Geometry: final body of the model. Coordinates: model frame, mm. A direction names the side the tool comes from. Give positions to 0.01 mm unless a question says otherwise; leave off trailing zeros. Write each loop counter-clockwise with the first axis right and the second up, starting at its lowest first coordinate (ties: lowest second). Pieces come first, ordered by that corner, then holes.
```python
from build123d import *

# Parameters (mm, degrees)
CYLINDER027_R     = 2
CYLINDER027_DEPTH = 10
CYLINDER025_R     = 2
CYLINDER025_DEPTH = 10
CYLINDER024_R     = 2
CYLINDER024_DEPTH = 10
CYLINDER023_R     = 4
CYLINDER023_DEPTH = 60
CYLINDER028_R     = 7.5
CYLINDER028_DEPTH = 40
BOX005_W          = 25
BOX005_H          = 25
BOX005_DEPTH      = 5.2


with BuildPart() as cylinder027:
    # Cylinder027 → Cylinder027 (new body)
    with BuildSketch(Plane(origin=(21, 4, -2), x_dir=(1, 0, 0), z_dir=(0, 0, 1))):
        Circle(CYLINDER027_R)
    extrude(amount=CYLINDER027_DEPTH)


with BuildPart() as cylinder025:
    # Cylinder025 → Cylinder025 (new body)
    with BuildSketch(Plane(origin=(4, 21, -2), x_dir=(1, 0, 0), z_dir=(0, 0, 1))):
        Circle(CYLINDER025_R)
    extrude(amount=CYLINDER025_DEPTH)


with BuildPart() as cylinder024:
    # Cylinder024 → Cylinder024 (new body)
    with BuildSketch(Plane(origin=(4, 4, -2), x_dir=(1, 0, 0), z_dir=(0, 0, 1))):
        Circle(CYLINDER024_R)
    extrude(amount=CYLINDER024_DEPTH)


with BuildPart() as cylinder023:
    # Cylinder023 → Cylinder023 (new body)
    with BuildSketch(Plane(origin=(12.5, 12.5, -7), x_dir=(1, 0, 0), z_dir=(0, 0, 1))):
        Circle(CYLINDER023_R)
    extrude(amount=CYLINDER023_DEPTH)


with BuildPart() as cylinder028:
    # Cylinder028 → Cylinder028 (new body)
    with BuildSketch(Plane(origin=(12.5, 12.5, 5), x_dir=(1, 0, 0), z_dir=(0, 0, 1))):
        Circle(CYLINDER028_R)
    extrude(amount=CYLINDER028_DEPTH)


with BuildPart() as cut026:
    # Box005 → Box005 (new body)
    with BuildSketch(Plane.XY):
        with Locations((12.5, 12.5)):
            Rectangle(BOX005_W, BOX005_H)
    extrude(amount=BOX005_DEPTH)

    # Fusion006: union Cylinder028
    add(cylinder028.part)

    # Cut027: cut Cylinder023
    add(cylinder023.part, mode=Mode.SUBTRACT)

    # Cut028: cut Cylinder024
    add(cylinder024.part, mode=Mode.SUBTRACT)

    # Cut025: cut Cylinder025
    add(cylinder025.part, mode=Mode.SUBTRACT)

    # Cut026: cut Cylinder027
    add(cylinder027.part, mode=Mode.SUBTRACT)


solid = cut026.part
```
Item 1: Section D-D, the plane z = 7.5. Return the cut outline in (x, y), plus the area to 3 significant figures.
Found:
outline: circle Ø15 at (12.5, 12.5); hole circle Ø8 at (12.5, 12.5)
area: 126 mm2
Item 2: Pull-direction query (X, two-part tool) for faces 1 (the face through (11.979, 16.466, 22.185)), 2 (the face through (12, 25, 3)), 3 (the face through (0, 12, 3)); classes: +X half, -X half, draft (parallel to the pull), parting line (faces both ways), or undercut.
Found:
face 1: undercut
face 2: draft
face 3: -X half
Item 3: Section C-C, the plane y = 21. Return the cut outline in (x, z).
Found:
outline: (0, 0) - (2, 0) - (2, 5.2) - (0, 5.2) - close; (6, 0) - (25, 0) - (25, 5.2) - (6, 5.2) - close
Item 4: Line query: L1, parallel to Y at x = 4, z = 4; L2, parallel to X at y = 12.5, z = 15.5. Output: solid intervals per line, ascending.
Found:
L1: y = 0 to 2, 6 to 19, 23 to 25
L2: x = 5 to 8.5, 16.5 to 20
Item 5: Section A-A, the plane x = 12.5. Return the cut outline in (y, z), plus the area to 3 significant figures.
Found:
outline: (0, 0) - (8.5, 0) - (8.5, 45) - (5, 45) - (5, 5.2) - (0, 5.2) - close; (16.5, 0) - (25, 0) - (25, 5.2) - (20, 5.2) - (20, 45) - (16.5, 45) - close
area: 367 mm2
Item 6: Section B-B, the plane y = 4. Return the cut outline in (x, z), plus the area to 3 significant figures.
Found:
outline: (0, 0) - (2, 0) - (2, 5.2) - (0, 5.2) - close; (6, 0) - (19, 0) - (19, 5.2) - (6, 5.2) - close; (23, 0) - (25, 0) - (25, 5.2) - (23, 5.2) - close
area: 88.4 mm2
Item 7: Reachability of faces 4 (the face through (10.87, 5.18, 24.82)), 5 (the face through (19.4, 2.8, 2.6)) from +Z, -Z, +X, -X, +Y, -Y: full face, straight path, thin tool, end or side. Return the list, or none.
Found:
face 4: +Z
face 5: +Z, -Z
Item 8: Pin query (flat end, axial travel): pin 1 Ø3 at (x, z) = (20, 12.5) entering from +Y; pin 2 Ø4 at (x, y) = (22.5, 22) entering from +Z; pin 3 Ø2 at (y, z) = (8, 11.5) entering from +X. Return the tip coordinate at first contact, or that it passes through.
Found:
pin 1: stops at y = 17
pin 2: stops at z = 5.2
pin 3: stops at x = 19.13
